The listing builds one solid part. Answer for the finished solid, in the listing's coordinates (mm). Face numbers are marked on the shaded views. Give positions to 0.01 mm unless a question says otherwise; leave off trailing zeros. Order: outer loops, then holes, each group sorted by start corner. A loop starts at its lowest first (then second) coordinate and runs counter-clockwise, first axis right, second up. Notation, with made-up numbers: (-13, 72.25) -> (14, 72.25) arc R20 ccw to (14, 99.25) -> close; hole circle Ø5 at (13.25, -27). An arc over 180 degrees is marked (long way). One line per question, with ' | ' between items. Start each with the question number.
```python
from build123d import *

# Parameters (mm, degrees)
F0_R            = 42.5
F1_DEPTH        = 85
F3_DEPTH        = 85.001
F3_COPIES_COUNT = 3


# Not quite as in the source:
# - a pattern or mirror of a feature is missing from the dataset's text; its kind, count and spacing are read off the source's solid


with BuildPart() as f1:
    # F0 (on Top) → F1 (new body)
    with BuildSketch(Plane.XY):
        Circle(F0_R)
    extrude(amount=F1_DEPTH)

    # F2 (on face) → F3 (cut, through all)
    with BuildSketch(Plane.XY.offset(85)):
        with BuildLine():
            Line((15, -2.05), (18.0782255906, -2.05))
            ThreePointArc((18.0782255906, -2.05), (40.1125, 0), (18.0782255906, 2.05))
            Line((18.0782255906, 2.05), (15, 2.05))
            Line((15, 2.05), (15, -2.05))
        make_face()
    f3 = extrude(amount=-F3_DEPTH, mode=Mode.SUBTRACT)

    # F3_copies: F3 ×3 about axis
    f3_copies_axis = Axis((0, 0, 0), (0, 0, 1))
    for i in range(1, F3_COPIES_COUNT):
        add(f3.rotate(f3_copies_axis, i * 360 / F3_COPIES_COUNT), mode=Mode.SUBTRACT)


solid = f1.part
```
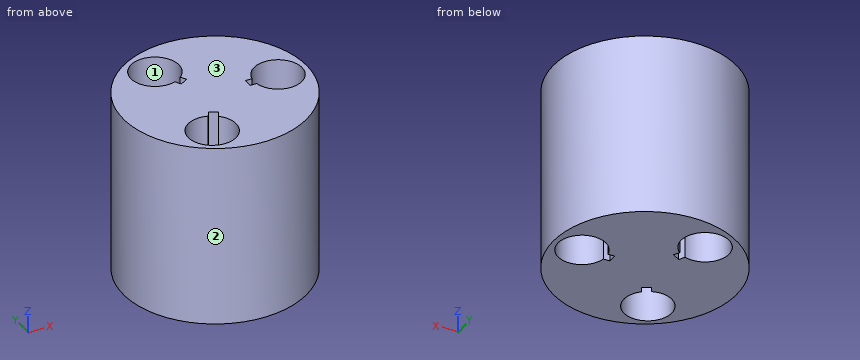
(1) The part is cut by section D-D on x = 29. Determine the outline of the cut face in (y, z), plus the area to 3 significant figures.
(2) The part is cut by section A-A on y = 0. Determine the outline of the cut face in (x, z), plus the area to 3 significant figures.
(3) Given P1, Ø1.5, axis at x = 17, z = 26.5, coming from the +Y side; P2, Ø10, axis at x = 1.5, z = 71.5, coming from the +Y side; P3, Ø10, axis at x = -16.5, z = 65.5, coming from the +Y side; P4, Ø8, axis at x = -20.5, y = -2, coming from the -Z side, each flat-ended and moving along its own axis, determine where each tip first touches the part or whether it passes through.
(4) Determine the mould class of the marked faces 1, 2 and 3 for opening direction X: pulls with the +X half, pulls with the -X half, needs draft (parallel to the pull), parting line crosses it, or undercut.
(5) The part is cut by section C-C on z = 24. State how many separate pieces and enclosed holes the cut face has, plus the area to 3 significant figures.
(6) The part is cut by section B-B on x = -12. Determine the outline of the cut face in (y, z), plus the area to 3 significant figures.
(7) Consider line 1 (Y direction, x = -14.5, z = 42); line 2 (Y direction, x = -12, z = 5); line 3 (X direction, y = -4.5, z = 59). Determine where each line is inside the solid, lowest interval first.
Result sheet:
1) outline: (-31.07, 0) -> (-11.11, 0) -> (-11.11, 85) -> (-31.07, 85) -> close; (11.11, 0) -> (31.07, 0) -> (31.07, 85) -> (11.11, 85) -> close | area: 3,390 mm^2
2) outline: (-42.5, 0) -> (15, 0) -> (15, 85) -> (-42.5, 85) -> close; (40.11, 0) -> (42.5, 0) -> (42.5, 85) -> (40.11, 85) -> close | area: 5,090 mm^2
3) P1: stops at y = 39.27 | P2: stops at y = 42.5 | P3: stops at y = 40.91 | P4: stops at z = 0
4) face 1: undercut | face 2: parting line crosses it | face 3: needs draft
5) separate pieces: 1 | enclosed holes: 3 | area: 4,470 mm^2
6) outline: (-40.77, 0) -> (-35.94, 0) -> (-35.94, 85) -> (-40.77, 85) -> close; (-14.29, 0) -> (14.29, 0) -> (14.29, 85) -> (-14.29, 85) -> close; (35.94, 0) -> (40.77, 0) -> (40.77, 85) -> (35.94, 85) -> close | area: 3,250 mm^2
7) line 1: y = -39.95 to -36.23, -14 to 14, 36.23 to 39.95 | line 2: y = -40.77 to -35.94, -14.29 to 14.29, 35.94 to 40.77 | line 3: x = -42.26 to 18.84, 39.16 to 42.26
